```python
from build123d import *

# Parameters (mm, degrees)
BOSS_EXTRUDE1_DEPTH      = 15
BOSS_EXTRUDE1_DEPTH_BACK = 15
SKETCH2_R                = 2
CUT_EXTRUDE1_DEPTH       = 24
SKETCH3_R                = 2
CUT_EXTRUDE2_DEPTH       = 24
SKETCH6_R                = 2.9765625
CUT_EXTRUDE4_DEPTH       = 73.013836648


with BuildPart() as part:
    # Sketch1 → Boss-Extrude1 (new, two sides: drawn at the far end of the back side and taken through both)
    with BuildSketch(Plane.XY.offset(-BOSS_EXTRUDE1_DEPTH_BACK)):
        with BuildLine():
            Line((5, -49.80458146), (-5, -49.80458146))
            Line((-5, -49.80458146), (-5, -49.552964941))
            ThreePointArc((-5, -49.552964941), (-6.59229192, -49.366365287), (-8.177753112, -49.128613744))
            ThreePointArc((-8.177753112, -49.128613744), (-10.602641493, -48.324877157), (-12.666415249, -46.819249696))
            Line((-12.666415249, -46.819249696), (-32.231963719, -27.253701226))
            ThreePointArc((-32.231963719, -27.253701226), (-32.231963719, 32.231963719), (27.253701226, 32.231963719))
            Line((27.253701226, 32.231963719), (46.819249696, 12.666415249))
            ThreePointArc((46.819249696, 12.666415249), (48.324877157, 10.602641493), (49.128613744, 8.177753112))
            ThreePointArc((49.128613744, 8.177753112), (49.366365287, 6.59229192), (49.552964941, 5))
            Line((49.552964941, 5), (49.80458146, 5))
            Line((49.80458146, 5), (49.80458146, -5))
            Line((49.80458146, -5), (49.552964941, -5))
            ThreePointArc((49.552964941, -5), (48.051135901, -13.099033286), (45.234948365, -20.839764414))
            Line((45.234948365, -20.839764414), (23.63175062, 0.763433331))
            Line((23.63175062, 0.763433331), (25.128673235, 2.260355947))
            Line((25.128673235, 2.260355947), (7.371511647, 20.017517534))
            ThreePointArc((7.371511647, 20.017517534), (-20.017517534, 20.017517534), (-20.017517534, -7.371511647))
            Line((-20.017517534, -7.371511647), (-2.260355947, -25.128673235))
            Line((-2.260355947, -25.128673235), (-0.763433331, -23.63175062))
            Line((-0.763433331, -23.63175062), (20.839764414, -45.234948365))
            ThreePointArc((20.839764414, -45.234948365), (13.099033286, -48.051135901), (5, -49.552964941))
            Line((5, -49.552964941), (5, -49.80458146))
        make_face()
    extrude(amount=BOSS_EXTRUDE1_DEPTH + BOSS_EXTRUDE1_DEPTH_BACK)

    # Sketch2 → Cut-Extrude1 (cut)
    with BuildSketch(Plane(origin=(0, -49.80458146, 0), x_dir=(1, 0, 0), z_dir=(0, 1, 0))):
        with Locations(Location((0, 0, 0), (0, 0, 314.805212022))):
            Circle(SKETCH2_R)
    extrude(amount=CUT_EXTRUDE1_DEPTH, mode=Mode.SUBTRACT)

    # Sketch3 → Cut-Extrude2 (cut)
    with BuildSketch(Plane(origin=(49.80458146, 0, 0), x_dir=(0, 0, -1), z_dir=(1, 0, 0))):
        Circle(SKETCH3_R)
    extrude(amount=-CUT_EXTRUDE2_DEPTH, mode=Mode.SUBTRACT)

    # Sketch6 → Cut-Extrude4 (cut, through all)
    with BuildSketch(Plane.XY):
        with Locations((-9.058666579, -33.80740392)):
            Circle(SKETCH6_R)
        with Locations((-35, 0)):
            Circle(SKETCH6_R)
        with Locations(Location((0, 35, 0), (0, 0, 180))):
            Circle(SKETCH6_R)
        with Locations(Location((33.80740392, 9.058666579, 0), (0, 0, 180))):
            Circle(SKETCH6_R)
    extrude(amount=CUT_EXTRUDE4_DEPTH, mode=Mode.SUBTRACT)


solid = part.part
```
The listing builds one solid part. Answer for the finished solid, in the listing's coordinates (mm). A direction names the side the tool comes from. Coordinates: 2 decimals unless noted, no trailing zeros. Write each loop counter-clockwise with the first axis right and the second up, starting at its lowest first coordinate (ties: lowest second). Pieces come first, ordered by that corner, then holes. Notation, with made-up numbers: M 42.5,-30.5 L 87.5,-30.5 A32 ccw 87.5,0.5 Z; hole C 78,-20.75 d7. An arc over 180 degrees is marked long. Use a Markdown table: item, result. Add a question column.
1. Section B-B (y = -18) is taken. Give the vertices of the cut face in (x, z).
2. Section D-D (x = 38) is taken. Give the vertices of the cut face in (y, z), plus the area to 3 significant figures.
3. Which of the six approach directions +Z, -Z, +X, -X, +Y, -Y give full straight-line access (tool end or side, diameter ignored) to faces 1 (the flat face through (0, -25.805, 0)), 2 (the flat face through (9.887, -34.282, -0.21)), 3 (the flat face through (-9, -34, 0)), 4 (the cylindrical face through (38, -2, 0))?
4. Given P1, Ø6.5, axis at x = 0, z = 0, coming from the +Y side; P2, Ø2, axis at x = -9.5, z = 4.5, coming from the -Y side; P3, Ø5, axis at y = -7.5, z = 1.5, coming from the -X side; P4, Ø3, axis at x = -34.5, y = -1, coming from the +Z side, each flat-ended and moving along its own axis, determine where each tip first touches the part or whether it passes through.
5. For a pull along Y with two mould halves and no side action, classify faces 5 (the flat face through (49.805, -2.2, -0.2)), 6 (the cylindrical face through (13.21, -48.02, -0.21)), 7 (the flat face through (-11.26, -16.13, -0.21)) as +Y half, -Y half, draft (parallel to the pull), parting line (faces both ways), or undercut.
6. Section A-A (z = -5.5) is taken. Give the vertices of the cut face in (x, y).
7. Straight lines are drawn through the part: line 1 along Y through (x, z) = (-1, 6.5); line 2 along Y through (x, z) = (-24, -9.5); line 3 along X through (y, z) = (-41, 0). For each, find the intervals that lie inside material, in ascending order. Write a range as [from, to].
8. Section C-C (x = -35) is taken. Give the vertices of the cut face in (y, z), plus the area to 3 significant figures.
Data:
| question | item | result |
|---|---|---|
| 1 | outline | M -39.22,-15 L -9.39,-15 L -9.39,15 L -39.22,15 Z; M 42.4,-15 L 46.44,-15 L 46.44,15 L 42.4,15 Z |
| 2 | outline | M -13.6,-15 L 21.49,-15 L 21.49,15 L -13.6,15 Z; hole C 0,0 d4 |
| 2 | area | 1,040 mm2 |
| 3 | face 1 | -Y |
| 3 | face 2 | +Z, -Z, +X |
| 3 | face 3 | +Z |
| 3 | face 4 | +X |
| 4 | P1 | stops at y = 44.55 |
| 4 | P2 | stops at y = -49.07 |
| 4 | P3 | stops at x = -43.88 |
| 4 | P4 | stops at z = 0 |
| 5 | face 5 | draft |
| 5 | face 6 | -Y half |
| 5 | face 7 | undercut |
| 6 | outline | M -32.23,-27.25 L -12.67,-46.82 A8.27 ccw -8.18,-49.13 A49.8 ccw -5,-49.55 L -5,-49.8 L 5,-49.8 L 5,-49.55 A49.8 ccw 20.84,-45.23 L -0.76,-23.63 L -2.26,-25.13 L -20.02,-7.37 A19.37 cw 7.37,20.02 L 25.13,2.26 L 23.63,0.76 L 45.23,-20.84 A49.8 ccw 49.55,-5 L 49.8,-5 L 49.8,5 L 49.55,5 A49.8 ccw 49.13,8.18 A8.27 ccw 46.82,12.67 L 27.25,32.23 A42.06 ccw Z |
| 7 | line 1 | y = [-49.8, -23.87], [24.94, 32.2], [37.8, 44.53] |
| 7 | line 2 | y = [-35.49, -1.59], [14.24, 38.64] |
| 7 | line 3 | x = [-18.49, -2], [2, 16.6] |
| 8 | outline | M -24.2,-15 L 29.18,-15 L 29.18,15 L 2.98,15 L 2.98,0 L -2.98,0 L -2.98,15 L -24.2,15 Z |
| 8 | area | 1,510 mm2 |
